Can you work these out from the model? Positions are in its coordinate system, mm. Round coordinates to 2 decimals unless told otherwise and drop trailing zeros. Write each loop counter-clockwise with the first axis right and the second up, starting at its lowest first coordinate (ties: lowest second). Pieces come first, ordered by that corner, then holes. Notation, with made-up numbers: (-17.75, 76.5) -> (18.25, 76.5) arc R9 cw to (18.25, 87.5) -> close; hole circle Ø6 at (-17, 51.25). An arc over 180 degrees is marked (long way). Write item = value, one per line. Start each with the question number.
1) I'm going to push flat-ended pins straight in: pin 1 (8.5 mm diameter, centred on x = 60.49, z = -116.1, fed in from -Y); pin 2 (2 mm diameter, centred on y = 1, z = -25, fed in from -X); pin 3 (1 mm diameter, centred on y = 4.5, z = -21, fed in from -X). Where does each tip first touch, or does it pass through?
2) Imagine slicing it at C-C, the plane y = 3.65. State how many separate pieces and enclosed holes the cut face has, then the cut area to 3 significant figures.
3) Imagine slicing it at A-A, the plane x = 66. Please give me the cut outline in (y, z), then the cut area to 3 significant figures.
4) If I drill on line 1 (Z direction, x = 28, y = 2.45); line 2 (Z direction, x = 29.5, y = 3.2); line 3 (X direction, y = 3.45, z = -61.5), over which ranges is the centre line in solid material (lowest first)?
5) Imagine slicing it at B-B, the plane z = -79. Please give me the cut outline in (x, y), then the cut area to 3 significant figures.
6) Imagine slicing it at D-D, the plane x = -63. Please give me the cut outline in (y, z), then the cut area to 3 significant figures.
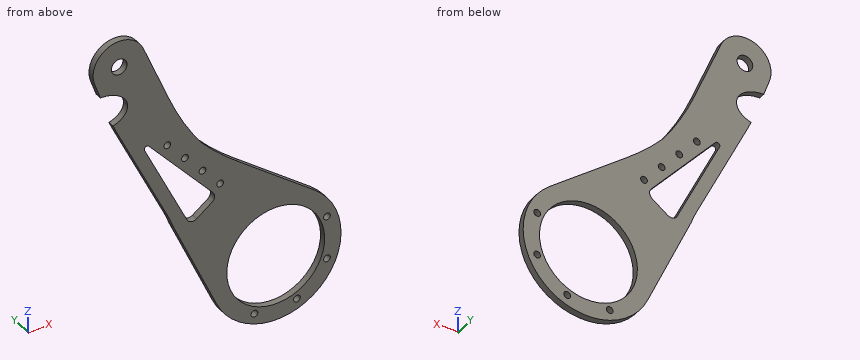
from build123d import *

# Parameters (mm, degrees)
SKETCH_4_R          = 6
SKETCH_4_R_2        = 37.5
SKETCH_4_R_3        = 2.6
EXTRUDE_1_DEPTH     = 5
SKETCH_5_R          = 2.6
CUT_EXTRUDE_1_DEPTH = 5


with BuildPart() as part:
    # 草图4 → 凸台-拉伸1 (new body)
    with BuildSketch(Plane(origin=(0, 0, 0), x_dir=(1, 0, 0), z_dir=(0, 1, 0))):
        with BuildLine():
            Line((-1.187051208, 97.756382931), (-34.399966732, 25.661973505))
            ThreePointArc((-34.399966732, 25.661973505), (-36.436671314, 20.514211828), (-38.755127266, 15.487047832))
            Line((-38.755127266, 15.487047832), (-76.702239109, -61.142758857))
            ThreePointArc((-76.702239109, -61.142758857), (-78.581308529, -65.042906811), (-80.375519882, -68.982813099))
            add(Edge.make_bspline(
                [(-90.080878885, -94.318710442), (-73.900652668, -94.557787877), (-69.815317221, -83.892995419), (-65.729981774, -73.228202961), (-80.375519882, -68.982813099)],
                knots=[1.469085418, 1.469085418, 1.469085418, 2.850930512, 2.850930512, 4.232775606, 4.232775606, 4.232775606], degree=2, weights=[1, 0.770658452, 1, 0.770658452, 1]))
            Line((-90.080878885, -94.318710442), (-94.447090172, -106.314777361))
            ThreePointArc((-94.447090172, -106.314777361), (-82.99415066, -131.759238863), (-57.252299544, -120.991344654))
            Line((-57.252299544, -120.991344654), (-37.073490807, -73.607319444))
            ThreePointArc((-37.073490807, -73.607319444), (-26.275484562, -51.979867968), (-12.947104361, -31.813116187))
            ThreePointArc((-12.947104361, -31.813116187), (1.038966567, -18.243877447), (16.279183802, -6.100146611))
            Line((16.279183802, -6.100146611), (73.992008997, 36.661223905))
            ThreePointArc((73.992008997, 36.661223905), (75.759044699, 115.638002674), (-1.187051208, 97.756382931))
        make_face()
        with Locations(Location((-75.653237756, -113.155180227, 0), (0, 0, 270))):
            Circle(SKETCH_4_R, mode=Mode.SUBTRACT)
        with Locations(Location((44.225629177, 76.835377691, 0), (0, 0, 270))):
            Circle(SKETCH_4_R_2, mode=Mode.SUBTRACT)
        with Locations(Location((-38.804653771, -38.995185245, 0), (0, 0, 270))):
            Circle(SKETCH_4_R_3, mode=Mode.SUBTRACT)
        with Locations(Location((-11.835571633, -9.45422032, 0), (0, 0, 270))):
            Circle(SKETCH_4_R_3, mode=Mode.SUBTRACT)
        with Locations(Location((-25.320112702, -24.224702783, 0), (0, 0, 270))):
            Circle(SKETCH_4_R_3, mode=Mode.SUBTRACT)
        with Locations(Location((1.648969436, 5.316262142, 0), (0, 0, 270))):
            Circle(SKETCH_4_R_3, mode=Mode.SUBTRACT)
        with BuildLine():
            Line((-23.760910885, 24.444490758), (-56.249753951, -41.162972966))
            ThreePointArc((-56.249753951, -41.162972966), (-55.586524246, -43.701342116), (-52.980423674, -43.398965873))
            Line((-52.980423674, -43.398965873), (-3.889961488, 10.372965042))
            ThreePointArc((-3.889961488, 10.372965042), (-2.608449448, 14.252041571), (-4.647570443, 17.792026514))
            Line((-4.647570443, 17.792026514), (-16.345194148, 26.273569961))
            ThreePointArc((-16.345194148, 26.273569961), (-20.477567373, 27.080159725), (-23.760910885, 24.444490758))
        make_face(mode=Mode.SUBTRACT)
    extrude(amount=EXTRUDE_1_DEPTH)

    # 草图5 → 切除-拉伸1 (cut)
    with BuildSketch(Plane(origin=(0, 5, 0), x_dir=(1, 0, 0), z_dir=(0, 1, 0))):
        with Locations(Location((60.489675053, 116.100257823, 0), (0, 0, 270))):
            Circle(SKETCH_5_R)
        with Locations(Location((83.490509309, 93.099423567, 0), (0, 0, 270))):
            Circle(SKETCH_5_R)
        with Locations(Location((83.490509309, 60.571331816, 0), (0, 0, 270))):
            Circle(SKETCH_5_R)
        with Locations(Location((27.961583302, 116.100257823, 0), (0, 0, 270))):
            Circle(SKETCH_5_R)
    extrude(amount=-CUT_EXTRUDE_1_DEPTH, mode=Mode.SUBTRACT)


solid = part.part
Reported:
q1.pin_1 = 0
q1.pin_2 = -35.02
q1.pin_3 = -36.44
q2.separate_pieces = 1
q2.enclosed_holes = 11
q2.area = 11,500 mm²
q3.outline = (0, -121.85) -> (5, -121.85) -> (5, -107.37) -> (0, -107.37) -> close; (0, -46.3) -> (5, -46.3) -> (5, -30.74) -> (0, -30.74) -> close
q3.area = 150 mm²
q4.line_1 = -124.13 to -118.7, -113.5 to -110.64, -43.03 to -2.58
q4.line_2 = -124.62 to -118.2, -114 to -111.32, -42.35 to -3.7
q4.line_3 = -17.89 to 10, 78.45 to 81.06, 85.92 to 91.82
q5.outline = (-9.83, 0) -> (6.79, 0) -> (6.79, 5) -> (-9.83, 5) -> close; (81.66, 0) -> (94.18, 0) -> (94.18, 5) -> (81.66, 5) -> close
q5.area = 146 mm²
q6.outline = (0, 33.47) -> (5, 33.47) -> (5, 128.64) -> (0, 128.64) -> close
q6.area = 476 mm²
